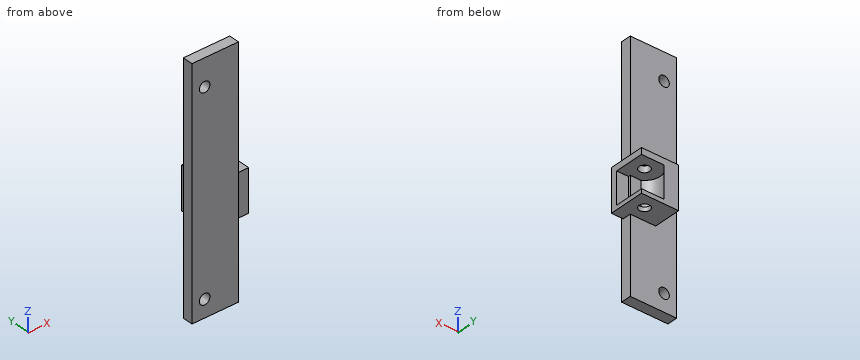
```python
from build123d import *

# Parameters (mm, degrees)
BOSS_EXTRUDE1_DEPTH      = 21.59
SKETCH2_W                = 22.352
SKETCH2_H                = 21.59
SKETCH2_R                = 3.175
BOSS_EXTRUDE2_DEPTH      = 3.81
BOSS_EXTRUDE3_START      = -2.54
SKETCH3_R                = 3.175
BOSS_EXTRUDE3_DEPTH      = 2.54
BOSS_EXTRUDE4_DEPTH      = 1.164777
BOSS_EXTRUDE4_DEPTH_BACK = 5.08
SKETCH4_W                = 27.94
SKETCH4_H                = 144.78
SKETCH4_R                = 3.175


with BuildPart() as part:
    # Sketch1 → Boss-Extrude1 (new body)
    with BuildSketch(Plane.XY):
        with BuildLine():
            Line((-792.583825879, 92.376177143), (-792.583825879, 96.160777143))
            Line((-792.583825879, 96.160777143), (-801.338321143, 96.160777143))
            ThreePointArc((-801.338321143, 96.160777143), (-803.772947911, 96.477182381), (-806.045825879, 97.405377143))
            ThreePointArc((-806.045825879, 97.405377143), (-810.863321143, 105.685777143), (-806.045825879, 113.966177143))
            Line((-806.045825879, 113.966177143), (-814.935825879, 113.966177143))
            Line((-814.935825879, 113.966177143), (-814.935825879, 92.376177143))
            Line((-814.935825879, 92.376177143), (-792.583825879, 92.376177143))
        make_face()
    extrude(amount=-BOSS_EXTRUDE1_DEPTH)

    # Sketch2 → Boss-Extrude2 (add)
    with BuildSketch(Plane.XY):
        with Locations((-803.759825879, 103.171177143)):
            Rectangle(SKETCH2_W, SKETCH2_H)
        with Locations(Location((-801.338321143, 105.685777143, 0), (0, 0, 180))):
            Circle(SKETCH2_R, mode=Mode.SUBTRACT)
    extrude(amount=BOSS_EXTRUDE2_DEPTH)

    # Sketch3 → Boss-Extrude3 (add)
    with BuildSketch(Plane(origin=(0, 0, -21.59), x_dir=(-1, 0, 0), z_dir=(0, 0, -1)).offset(BOSS_EXTRUDE3_START)):
        with BuildLine():
            Line((792.583825879, 113.966177143), (792.583825879, 96.160777143))
            Line((792.583825879, 96.160777143), (801.338321143, 96.160777143))
            ThreePointArc((801.338321143, 96.160777143), (810.546915906, 103.251150375), (806.045825879, 113.966177143))
            Line((806.045825879, 113.966177143), (792.583825879, 113.966177143))
        make_face()
        with Locations((801.338321143, 105.685777143)):
            Circle(SKETCH3_R, mode=Mode.SUBTRACT)
    extrude(amount=BOSS_EXTRUDE3_DEPTH)

    # Sketch4 → Boss-Extrude4 (add, two sides: drawn at the far end of the back side and taken through both)
    with BuildSketch(Plane.XZ.offset(-92.376177143).offset(-BOSS_EXTRUDE4_DEPTH_BACK)):
        with Locations((-813.665825879, 5.08)):
            Rectangle(SKETCH4_W, SKETCH4_H)
        with Locations(Location((-820.039, -56.765714286, 0), (0, 0, 270))):
            Circle(SKETCH4_R, mode=Mode.SUBTRACT)
        with Locations(Location((-820.039, 61.162857143, 0), (0, 0, 270))):
            Circle(SKETCH4_R, mode=Mode.SUBTRACT)
    extrude(amount=BOSS_EXTRUDE4_DEPTH + BOSS_EXTRUDE4_DEPTH_BACK)


solid = part.part
```
Geometry check sheet. Reference: the model listing, model coordinates, mm. Coordinates: 2 decimals unless noted, no trailing zeros. Loops run counter-clockwise (first coordinate to the right, second up) from the corner with the lowest first, then second, coordinate; pieces in that order, holes last.
Item 1: Go/stop test with flat-tipped pins: pin 1 Ø2 at (x, z) = (-796, -3.5) entering from -Y; pin 2 Ø1.9 at (x, z) = (-802, -5) entering from +Y; pin 3 Ø5.5 at (x, y) = (-801.34, 105.69) entering from -Z; pin 4 Ø8 at (y, z) = (97.5, 23.5) entering from +X. Record where each tip stops, or that it passes through.
Item 2: Sectioned sample at C-C, the plane x = -822. Record the boundary of the cut face in (y, z), then the cut area to 3 significant figures.
Item 3: Thickness scan on line 1 (Z direction, x = -800, y = 99); line 2 (Y direction, x = -797, z = -19); line 3 (Z direction, x = -793.5, y = 96). Record the ranges inside material, lowest first.
Item 4: Sectioned sample at A-A, the plane x = -813.5. Record the boundary of the cut face in (y, z), then the cut area to 3 significant figures.
Item 5: Sectioned sample at D-D, the plane z = -40.5. Record the boundary of the cut face in (x, y), then the cut area to 3 significant figures.
Item 6: Sectioned sample at B-B, the plane z = -8. Record the boundary of the cut face in (x, y) (3 decimals).
Check result:
1. pin 1: stops at y = 92.38
1. pin 2: stops at y = 97.46
1. pin 3: passes through
1. pin 4: stops at x = -799.7
2. outline: (91.21, -67.31) - (97.46, -67.31) - (97.46, -59.26) - (91.21, -59.26) - close; (91.21, -54.27) - (97.46, -54.27) - (97.46, 58.67) - (91.21, 58.67) - close; (91.21, 63.66) - (97.46, 63.66) - (97.46, 77.47) - (91.21, 77.47) - close
2. area: 842 mm2
3. line 1: z = -21.59 to -19.05, 0 to 3.81
3. line 2: y = 92.38 to 96.16
3. line 3: z = -21.59 to 3.81
4. outline: (91.21, -67.31) - (97.46, -67.31) - (97.46, -21.59) - (113.97, -21.59) - (113.97, 3.81) - (97.46, 3.81) - (97.46, 77.47) - (91.21, 77.47) - close
4. area: 1,320 mm2
5. outline: (-827.64, 91.21) - (-799.7, 91.21) - (-799.7, 97.46) - (-827.64, 97.46) - close
5. area: 174 mm2
6. outline: (-827.636, 91.211) - (-799.696, 91.211) - (-799.696, 92.376) - (-792.584, 92.376) - (-792.584, 96.161) - (-799.696, 96.161) - (-799.696, 97.456) - (-806.134, 97.456) arc R9.525 cw to (-806.046, 113.966) - (-814.936, 113.966) - (-814.936, 97.456) - (-827.636, 97.456) - close
